For this review, take the finished solid that the model builds, in its own axes (mm). Face numbers are marked on the shaded views. A direction names the side the tool comes from. Round coordinates to 2 decimals unless told otherwise and drop trailing zeros. Order: outer loops, then holes, each group sorted by start corner. A loop starts at its lowest first (then second) coordinate and runs counter-clockwise, first axis right, second up. Notation, with made-up numbers: M 55.5,37.5 L 72.5,37.5 A20 ccw 72.5,49.5 Z; hole C 71,39 d3. An arc over 180 degrees is marked long. Answer in a Markdown table with one row per item. Add a question column.
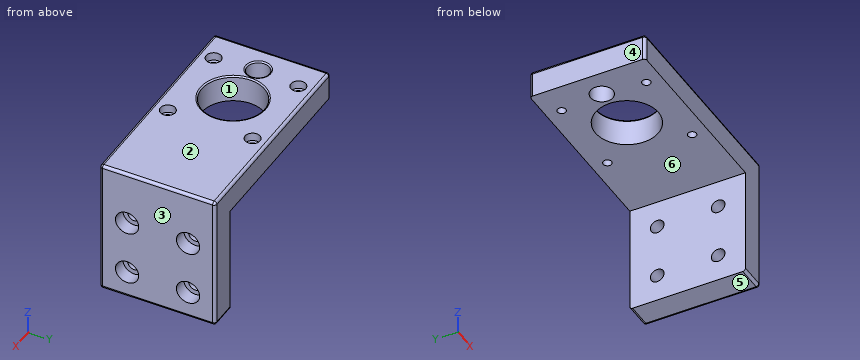
```python
from build123d import *

# Parameters (mm, degrees)
F0_W     = 42.3
F0_H     = 42.3
F0_R     = 2.75
F0_R_2   = 4.1
F0_R_3   = 11.5
F0_W_2   = 20
F0_W_3   = 5.5
F0_W_4   = 10
F0_R_4   = 1.55
F1_DEPTH = 10
F2_DEPTH = 40
F3_R     = 2.5
F4_DEPTH = 77.801
F3_R_2   = 4.25
F5_DEPTH = 5
F7_R     = 1
F8_R     = 0.5
F6_R     = 2.75
F6_R_2   = 1.55
F9_DEPTH = 3


with BuildPart() as f1:
    # F0 (on Top) → F1 (new body)
    with BuildSketch(Plane.XY):
        Rectangle(F0_W, F0_H)
        with Locations((-15.5, -15.5)):
            Circle(F0_R, mode=Mode.SUBTRACT)
        with Locations((15.5, -15.5)):
            Circle(F0_R, mode=Mode.SUBTRACT)
        with Locations((-17, 0)):
            Circle(F0_R_2, mode=Mode.SUBTRACT)
        Circle(F0_R_3, mode=Mode.SUBTRACT)
        with Locations((-15.5, 15.5)):
            Circle(F0_R, mode=Mode.SUBTRACT)
        with Locations((15.5, 15.5)):
            Circle(F0_R, mode=Mode.SUBTRACT)
        with Locations((31.15, 0)):
            Rectangle(F0_W_2, F0_H)
        with Locations((-23.9, 0)):
            Rectangle(F0_W_3, F0_H)
        with Locations((46.15, 0)):
            Rectangle(F0_W_4, F0_H)
        with Locations((-15.5, 15.5)):
            Circle(F0_R)
        with Locations((-15.5, 15.5)):
            Circle(F0_R_4, mode=Mode.SUBTRACT)
        with Locations((15.5, -15.5)):
            Circle(F0_R)
        with Locations((15.5, -15.5)):
            Circle(F0_R_4, mode=Mode.SUBTRACT)
        with Locations((-15.5, -15.5)):
            Circle(F0_R)
        with Locations((-15.5, -15.5)):
            Circle(F0_R_4, mode=Mode.SUBTRACT)
        with Locations((15.5, 15.5)):
            Circle(F0_R)
        with Locations((15.5, 15.5)):
            Circle(F0_R_4, mode=Mode.SUBTRACT)
    extrude(amount=F1_DEPTH)

    # F0 (on Top) → F2 (join)
    with BuildSketch(Plane.XY):
        with Locations((46.15, 0)):
            Rectangle(F0_W_4, F0_H)
    extrude(amount=-F2_DEPTH)

    # F3 (on face) → F4 (cut, through all)
    with BuildSketch(Plane.YZ.offset(51.15)):
        with Locations((-11.15, -10)):
            Circle(F3_R)
        with Locations((11.15, -10)):
            Circle(F3_R)
        with Locations((11.15, -30)):
            Circle(F3_R)
        with Locations((-11.15, -30)):
            Circle(F3_R)
    extrude(amount=-F4_DEPTH, mode=Mode.SUBTRACT)

    # F3 (on face) → F5 (cut)
    with BuildSketch(Plane.YZ.offset(51.15)):
        with Locations((-11.15, -10)):
            Circle(F3_R_2)
        with Locations((-11.15, -10)):
            Circle(F3_R, mode=Mode.SUBTRACT)
        with Locations((11.15, -10)):
            Circle(F3_R_2)
        with Locations((11.15, -10)):
            Circle(F3_R, mode=Mode.SUBTRACT)
        with Locations((11.15, -30)):
            Circle(F3_R_2)
        with Locations((11.15, -30)):
            Circle(F3_R, mode=Mode.SUBTRACT)
        with Locations((-11.15, -30)):
            Circle(F3_R_2)
        with Locations((-11.15, -30)):
            Circle(F3_R, mode=Mode.SUBTRACT)
    extrude(amount=-F5_DEPTH, mode=Mode.SUBTRACT)

    # F7
    f7_edges = [f1.edges().sort_by_distance(p)[0] for p in [
        (51.15, -21.15, -15),
        (51.15, 21.15, -15),
        (51.15, 0, -40),
        (51.15, 0, 10),
        (12.25, 21.15, 10),
        (12.25, -21.15, 10),
        (-26.65, 0, 10),
        (-26.65, 21.15, 5),
        (-26.65, -21.15, 5),
        (46.15, 21.15, -40),
        (46.15, -21.15, -40),
    ]]
    fillet(f7_edges, radius=F7_R)

    # F8
    f8_edges = [f1.edges().sort_by_distance(p)[0] for p in [
        (-21.1, 0, 10),
        (-11.5, 0, 10),
    ]]
    fillet(f8_edges, radius=F8_R)

    # F6 (on face) → F9 (cut)
    with BuildSketch(Plane.XY.offset(10)):
        with Locations((15.5, 15.5)):
            Circle(F6_R)
        with Locations((15.5, 15.5)):
            Circle(F6_R_2, mode=Mode.SUBTRACT)
        with Locations((15.5, -15.5)):
            Circle(F6_R)
        with Locations((15.5, -15.5)):
            Circle(F6_R_2, mode=Mode.SUBTRACT)
        with Locations((-15.5, -15.5)):
            Circle(F6_R)
        with Locations((-15.5, -15.5)):
            Circle(F6_R_2, mode=Mode.SUBTRACT)
        with Locations((-15.5, 15.5)):
            Circle(F6_R)
        with Locations((-15.5, 15.5)):
            Circle(F6_R_2, mode=Mode.SUBTRACT)
    extrude(amount=-F9_DEPTH, mode=Mode.SUBTRACT)


solid = f1.part
```
1. Consider section A-A on z = -30. Write out the cut boundary in (x, y).
2. Consider section B-B on y = 0. Write out the cut boundary in (x, z).
3. Consider section D-D on z = -19. Write out the cut boundary in (x, y), plus the area to 3 significant figures.
4. To check wall thickness, follow probe 1 along Z at (x, y) = (45, 11); probe 2 along Z at (x, y) = (-11.5, 16.5); probe 3 along X at (y, z) = (-15, 8). State the ranges of each line that lie inside material, in increasing order. Write a range as [from, to].
5. The part is to be moulded in two halves that separate along X. For the marked faces 1, 2, 3 and 4, say which applies: pulls with the +X half, pulls with the -X half, needs draft (parallel to the pull), parting line crosses it, or undercut.
6. Consider section C-C on x = 0. Write out the cut boundary in (y, z).
7. Clearance check with flat-ended pins moving along their axes: pin 1 Ø12 at (y, z) = (-2, -14.5) entering from -X; pin 2 Ø3 at (x, y) = (-15.5, 15.5) entering from +Z; pin 3 Ø1.5 at (x, y) = (40, -13) entering from -Z; pin 4 Ø3 at (x, y) = (-15, 14.5) entering from +Z. State where each tip first meets the part, or that it passes through.
8. For the marked faces 5 and 6, list the 3-axis set-ups (+Z, -Z, +X, -X, +Y, -Y) from which the entire face can be reached by the end or side of a thin tool; tool diameter is ignored.
Solved:
| question | item | result |
|---|---|---|
| 1 | outline | M 41.15,-21.15 L 50.15,-21.15 A1 ccw 51.15,-20.15 L 51.15,-15.4 L 46.15,-15.4 L 46.15,-13.65 L 41.15,-13.65 Z; M 41.15,-8.65 L 46.15,-8.65 L 46.15,-6.9 L 51.15,-6.9 L 51.15,6.9 L 46.15,6.9 L 46.15,8.65 L 41.15,8.65 Z; M 41.15,13.65 L 46.15,13.65 L 46.15,15.4 L 51.15,15.4 L 51.15,20.15 A1 ccw 50.15,21.15 L 41.15,21.15 Z |
| 2 | outline | M -26.65,0 L -21.1,0 L -21.1,9.5 A0.5 ccw -21.6,10 L -25.65,10 A1 ccw -26.65,9 Z; M -12.9,0 L -11.5,0 L -11.5,9.5 A0.5 ccw -12,10 L -12.4,10 A0.5 ccw -12.9,9.5 Z; M 11.5,0 L 41.15,0 L 41.15,-40 L 50.15,-40 A1 ccw 51.15,-39 L 51.15,9 A1 ccw 50.15,10 L 12,10 A0.5 ccw 11.5,9.5 Z |
| 3 | outline | M 41.15,-21.15 L 50.15,-21.15 A1 ccw 51.15,-20.15 L 51.15,20.15 A1 ccw 50.15,21.15 L 41.15,21.15 Z |
| 3 | area | 423 mm^2 |
| 4 | probe 1 | z = [-40, -32.5], [-27.5, -12.5], [-7.5, 10] |
| 4 | probe 2 | z = [0, 10] |
| 4 | probe 3 | x = [-26.65, -18.2], [-12.8, 12.8], [18.2, 51.15] |
| 5 | face 1 | undercut |
| 5 | face 2 | needs draft |
| 5 | face 3 | pulls with the +X half |
| 5 | face 4 | pulls with the -X half |
| 6 | outline | M -21.15,0 L -11.5,0 L -11.5,9.5 A0.5 ccw -12,10 L -20.15,10 A1 ccw -21.15,9 Z; M 11.5,0 L 21.15,0 L 21.15,9 A1 ccw 20.15,10 L 12,10 A0.5 ccw 11.5,9.5 Z |
| 7 | pin 1 | stops at x = 41.15 |
| 7 | pin 2 | passes through |
| 7 | pin 3 | stops at z = 0 |
| 7 | pin 4 | stops at z = 7 |
| 8 | face 5 | -Z, +X, -X, +Y, -Y |
| 8 | face 6 | -Z, -X, +Y, -Y |
